The listing builds one solid part. Answer for the finished solid, in the listing's coordinates (mm). Face numbers are marked on the shaded views. A direction names the side the tool comes from. Round coordinates to 2 decimals unless told otherwise and drop trailing zeros. Loops run counter-clockwise (first coordinate to the right, second up) from the corner with the lowest first, then second, coordinate; pieces in that order, holes last. Notation, with made-up numbers: (-9, -13.75) - (3, -13.75) arc R5 cw to (3, -8.75) - close; hole circle Ø9 at (66, -13). An arc over 180 degrees is marked (long way). Write item = value, one per line. Start each with the question number.
1) For a pull along Z with two mould halves and no side action, classify the marked faces 1, 2, 3 and 4 as released by +Z, released by -Z, zero draft, split by the parting line, or undercut.
2) Section A-A, the plane z = 0 is taken. Determine the outline of the cut face in (x, y).
3) Given pin 1 Ø12 at (x, z) = (41.5, 5) entering from -Y; pin 2 Ø4 at (x, z) = (24.5, -0.5) entering from -Y; pin 3 Ø5 at (x, y) = (4.5, -1.5) entering from +Z; pin 4 Ø0.9 at (y, z) = (3, 0) entering from -X, each flat-ended and moving along its own axis, determine where each tip first touches the part or whether it passes through.
4) Section D-D, the plane z = -5.5 is taken. Determine the outline of the cut face in (x, y).
5) Section B-B, the plane x = 4.5 is taken. Determine the outline of the cut face in (y, z), and give its area (3 significant figures).
6) A tool of negligible diameter and unlimited length cuts with its end or side. For the marked faces 5, 6, 7 and 8, from which of +Z, -Z, +X, -X, +Y, -Y can it reach the whole face along a straight path? Write none if from no direction.
7) Section C-C, the plane x = 10.5 is taken. Determine the outline of the cut face in (y, z), and give its area (3 significant figures).
8) Straight lines are drawn through the part: line 1 along X through (y, z) = (-1, 5.5); line 2 along X through (y, z) = (3.5, 1.5); line 3 along Z through (x, y) = (10, -1.25). For each, find the intervals that lie inside material, in ascending order.
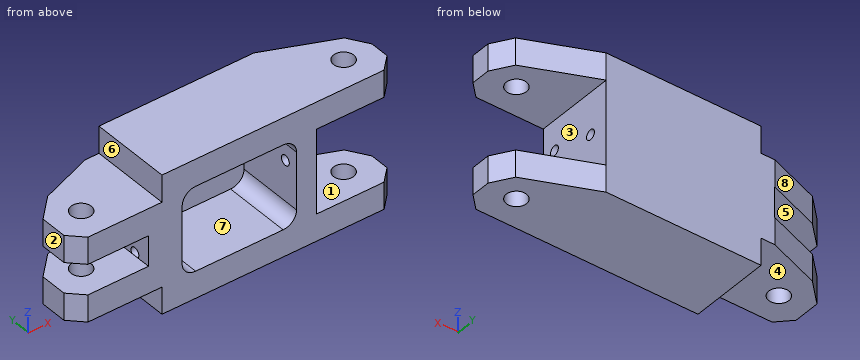
from build123d import *
from OCP.BRepFilletAPI import BRepFilletAPI_MakeChamfer

# Parameters (mm, degrees)
SKETCH_2_W            = 20.5
SKETCH_2_H            = 12
EXTRUDE_1_DEPTH       = 48
SKETCH_3_W            = 22
SKETCH_3_H            = 4.5
CUT_EXTRUDE_1_DEPTH   = 51.527838861
SKETCH_5_W            = 12
SKETCH_5_H            = 12.5
CUT_EXTRUDE_2_DEPTH   = 51.527838861
SKETCH_7_R            = 0.75
CUT_EXTRUDE_3_DEPTH   = 38.908607202
SKETCH_10_W           = 19.106520138
SKETCH_10_H           = 8.950699496
CUT_EXTRUDE_3_2_DEPTH = 51.527838861
SKETCH_11_R           = 1.5
CUT_EXTRUDE_6_DEPTH   = 52.110175112
SKETCH_9_R            = 1.5
CUT_EXTRUDE_5_DEPTH   = 53.538081427
SKETCH_12_R           = 0.75
CUT_EXTRUDE_4_DEPTH   = 12
CUT_EXTRUDE_7_DEPTH   = 53.538081427
CHAMFER_5_SIZE        = 2
CHAMFER_5_SIZE2       = 3.354740363
CHAMFER_6_SIZE        = 2
CHAMFER_6_SIZE2       = 2.1420728
SKETCH_14_R           = 0.75
CUT_EXTRUDE_5_2_DEPTH = 5
CUT_EXTRUDE_8_DEPTH   = 10


with BuildPart() as part:
    # Sketch 2 → Extrude 1 (new body)
    with BuildSketch(Plane(origin=(0, 0, 0), x_dir=(0, 0, -1), z_dir=(1, 0, 0))):
        Rectangle(SKETCH_2_W, SKETCH_2_H)
    extrude(amount=EXTRUDE_1_DEPTH)

    # Sketch 3 → Cut-Extrude 1 (cut, through all)
    with BuildSketch(Plane(origin=(0, 6, 0), x_dir=(1, 0, 0), z_dir=(0, 1, 0))):
        Rectangle(SKETCH_3_W, SKETCH_3_H)
    extrude(amount=-CUT_EXTRUDE_1_DEPTH, mode=Mode.SUBTRACT)

    # Sketch 5 → Cut-Extrude 2 (cut, through all)
    with BuildSketch(Plane(origin=(0, 6, 0), x_dir=(1, 0, 0), z_dir=(0, 1, 0))):
        with Locations((42, 0)):
            Rectangle(SKETCH_5_W, SKETCH_5_H)
    extrude(amount=-CUT_EXTRUDE_2_DEPTH, mode=Mode.SUBTRACT)

    # Sketch 7 → Cut-Extrude 3 (cut, through all)
    with BuildSketch(Plane(origin=(36, 0, 0), x_dir=(0, 0, -1), z_dir=(1, 0, 0))):
        with Locations((0, 3)):
            Circle(SKETCH_7_R)
    extrude(amount=-CUT_EXTRUDE_3_DEPTH, mode=Mode.SUBTRACT)

    # Sketch 10 → Cut-Extrude 3 2 (cut, through all)
    with BuildSketch(Plane(origin=(0, 6, 0), x_dir=(1, 0, 0), z_dir=(0, 1, 0))):
        with Locations((3.446739931, 10.725349748)):
            Rectangle(SKETCH_10_W, SKETCH_10_H)
        with Locations((3.446739931, -10.725349748)):
            Rectangle(SKETCH_10_W, SKETCH_10_H)
    extrude(amount=-CUT_EXTRUDE_3_2_DEPTH, mode=Mode.SUBTRACT)

    # Sketch 11 → Cut-Extrude 6 (cut, through all)
    with BuildSketch(Plane.XY.offset(6.25)):
        with Locations((4.5, -1.5)):
            Circle(SKETCH_11_R)
    extrude(amount=-CUT_EXTRUDE_6_DEPTH, mode=Mode.SUBTRACT)

    # Sketch 9 → Cut-Extrude 5 (cut, through all)
    with BuildSketch(Plane.XY.offset(10.25)):
        with Locations((43.5, -1.5)):
            Circle(SKETCH_9_R)
    extrude(amount=-CUT_EXTRUDE_5_DEPTH, mode=Mode.SUBTRACT)

    # Sketch 12 → Cut-Extrude 4 (cut)
    with BuildSketch(Plane.ZY.offset(-11)):
        with Locations((-1.791386219, -3.407348241)):
            Circle(SKETCH_12_R)
    extrude(amount=-CUT_EXTRUDE_4_DEPTH, mode=Mode.SUBTRACT)

    # Sketch 13 → Cut-Extrude 7 (cut, through all)
    with BuildSketch(Plane.XY.offset(10.25)):
        Polygon((10.95, 6), (0, 6), (0, 2), align=None)
        Polygon((48, 6), (48, 1), (36, 6), align=None)
    extrude(amount=-CUT_EXTRUDE_7_DEPTH, mode=Mode.SUBTRACT)

    # Chamfer 5: one chamfer whose edges measure the first distance from different faces: ONE call of the kernel's chamfer builder (chamfer() names one face for all edges)
    chamfer_5_edges_1 = [part.edges().sort_by_distance(p)[0] for p in [
        (0, 2, 4.25),
    ]]
    chamfer_5_side_1 = [part.faces().sort_by_distance(p)[0] for p in [
        (0, -2, 4.25),
    ]]
    chamfer_5_edges_2 = [part.edges().sort_by_distance(p)[0] for p in [
        (0, 2, -4.25),
    ]]
    chamfer_5_side_2 = [part.faces().sort_by_distance(p)[0] for p in [
        (0, -2, -4.25),
    ]]
    chamfer_5_edges_3 = [part.edges().sort_by_distance(p)[0] for p in [
        (48, -6, 8.25),
        (0, -6, -4.25),
        (48, -6, -8.25),
        (0, -6, 4.25),
    ]]
    chamfer_5 = BRepFilletAPI_MakeChamfer(part.part.solid().wrapped)
    for e in chamfer_5_edges_1:
        chamfer_5.Add(CHAMFER_5_SIZE, CHAMFER_5_SIZE2, e.wrapped, chamfer_5_side_1[0].wrapped)  # the first distance lies on this face
    for e in chamfer_5_edges_2:
        chamfer_5.Add(CHAMFER_5_SIZE, CHAMFER_5_SIZE2, e.wrapped, chamfer_5_side_2[0].wrapped)  # the first distance lies on this face
    for e in chamfer_5_edges_3:
        chamfer_5.Add(CHAMFER_5_SIZE, e.wrapped)
    add(Compound.cast(chamfer_5.Shape()), mode=Mode.REPLACE)

    # Chamfer 6: one chamfer whose edges measure the first distance from different faces: ONE call of the kernel's chamfer builder (chamfer() names one face for all edges)
    chamfer_6_edges_1 = [part.edges().sort_by_distance(p)[0] for p in [
        (48, 1, 8.25),
    ]]
    chamfer_6_side_1 = [part.faces().sort_by_distance(p)[0] for p in [
        (42, 3.5, 8.25),
    ]]
    chamfer_6_edges_2 = [part.edges().sort_by_distance(p)[0] for p in [
        (48, 1, -8.25),
    ]]
    chamfer_6_side_2 = [part.faces().sort_by_distance(p)[0] for p in [
        (42, 3.5, -8.25),
    ]]
    chamfer_6 = BRepFilletAPI_MakeChamfer(part.part.solid().wrapped)
    for e in chamfer_6_edges_1:
        chamfer_6.Add(CHAMFER_6_SIZE, CHAMFER_6_SIZE2, e.wrapped, chamfer_6_side_1[0].wrapped)  # the first distance lies on this face
    for e in chamfer_6_edges_2:
        chamfer_6.Add(CHAMFER_6_SIZE, CHAMFER_6_SIZE2, e.wrapped, chamfer_6_side_2[0].wrapped)  # the first distance lies on this face
    add(Compound.cast(chamfer_6.Shape()), mode=Mode.REPLACE)

    # Sketch 14 → Cut-Extrude 5 2 (cut)
    with BuildSketch(Plane(origin=(36, 0, 0), x_dir=(0, 0, -1), z_dir=(1, 0, 0))):
        with Locations((-1.767861063, -3.867641423)):
            Circle(SKETCH_14_R)
    extrude(amount=-CUT_EXTRUDE_5_2_DEPTH, mode=Mode.SUBTRACT)

    # Sketch 15 → Cut-Extrude 8 (cut)
    with BuildSketch(Plane.XZ.offset(6)):
        with BuildLine():
            Line((18, 6.25), (31, 6.25))
            ThreePointArc((31, 6.25), (32.414213562, 5.664213562), (33, 4.25))
            Line((33, 4.25), (33, -4.25))
            ThreePointArc((33, -4.25), (32.414213562, -5.664213562), (31, -6.25))
            Line((31, -6.25), (18, -6.25))
            ThreePointArc((18, -6.25), (16.585786438, -5.664213562), (16, -4.25))
            Line((16, -4.25), (16, 4.25))
            ThreePointArc((16, 4.25), (16.585786438, 5.664213562), (18, 6.25))
        make_face()
    extrude(amount=-CUT_EXTRUDE_8_DEPTH, mode=Mode.SUBTRACT)


solid = part.part
Geometry check:
q1.face_1 = undercut
q1.face_2 = zero draft
q1.face_3 = undercut
q1.face_4 = released by -Z
q2.outline = (11, -6) - (16, -6) - (16, 2.25) - (11, 2.25) - close; (11, 3.75) - (16, 3.75) - (16, 4) - (33, 4) - (33, 3.75) - (36, 3.75) - (36, 6) - (11, 6) - close; (33, -6) - (36, -6) - (36, 2.25) - (33, 2.25) - close
q3.pin_1 = -6
q3.pin_2 = 4
q3.pin_3 = 6.25
q3.pin_4 = through
q4.outline = (0, -4) - (2, -6) - (16.44, -6) - (16.44, 4) - (32.56, 4) - (32.56, -6) - (36, -6) - (36, 6) - (10.95, 6) - (3.15, 3.15) - (0, 0) - close; hole circle Ø3 at (4.5, -1.5)
q5.outline = (-6, -6.25) - (-3, -6.25) - (-3, -2.25) - (-6, -2.25) - close; (-6, 2.25) - (-3, 2.25) - (-3, 6.25) - (-6, 6.25) - close; (0, -6.25) - (3.64, -6.25) - (3.64, -2.25) - (0, -2.25) - close; (0, 2.25) - (3.64, 2.25) - (3.64, 6.25) - (0, 6.25) - close
q5.area = 53.2 mm2
q6.face_5 = -X, +Y, -Y
q6.face_6 = +Z, -X, +Y, -Y
q6.face_7 = -Y
q6.face_8 = +Z, -Z, -X, +Y
q7.outline = (-6, -6.25) - (5.84, -6.25) - (5.84, -2.25) - (-6, -2.25) - close; (-6, 2.25) - (5.84, 2.25) - (5.84, 6.25) - (-6, 6.25) - close
q7.area = 94.7 mm2
q8.line_1 = 0 to 3.09, 5.91 to 16.44, 32.56 to 36
q8.line_2 = 11 to 16, 33 to 36
q8.line_3 = -6.25 to -2.25, 2.25 to 6.25
